For this review, take the finished solid that the model builds, in its own axes (mm). Round coordinates to 2 decimals unless told otherwise and drop trailing zeros. Order: outer loops, then holes, each group sorted by start corner. A loop starts at its lowest first (then second) coordinate and runs counter-clockwise, first axis right, second up. Notation, with made-up numbers: M 77.25,24 L 130.25,24 A18 cw 130.25,41 Z; hole C -26.5,62.5 d6. An arc over 180 degrees is marked long. Use a Markdown table: item, result.
from build123d import *

# Parameters (mm, degrees)
SKETCH_1_W               = 86
SKETCH_1_H               = 86
EXTRUDE_1_DEPTH          = 2
FILLET_3_R               = 14
CUT_EXTRUDE_1_DEPTH      = 61.844062981
CUT_EXTRUDE_1_DEPTH_BACK = 61.844062981
SKETCH_2_R               = 5.5


with BuildPart() as part:
    # 草图1 → 凸台-拉伸1 (new body)
    with BuildSketch(Plane(origin=(0, 0, 0), x_dir=(1, 0, 0), z_dir=(0, 1, 0))):
        Rectangle(SKETCH_1_W, SKETCH_1_H)
    extrude(amount=EXTRUDE_1_DEPTH)

    # 圆角3
    fillet_3_edges = [part.edges().sort_by_distance(p)[0] for p in [
        (43, 1, 43),
        (-43, 1, 43),
        (-43, 1, -43),
        (43, 1, -43),
    ]]
    fillet(fillet_3_edges, radius=FILLET_3_R)

    # 草图2 → 切除-拉伸1 (cut, two sides: drawn at the far end of the back side and taken through both)
    with BuildSketch(Plane(origin=(0, 2, 0), x_dir=(1, 0, 0), z_dir=(0, 1, 0)).offset(-CUT_EXTRUDE_1_DEPTH_BACK)):
        with Locations(Location((-29, 29, 0), (0, 0, 270))):
            Circle(SKETCH_2_R)
        with Locations(Location((-29, -29, 0), (0, 0, 270))):
            Circle(SKETCH_2_R)
        with Locations(Location((29, -29, 0), (0, 0, 270))):
            Circle(SKETCH_2_R)
        with Locations(Location((29, 29, 0), (0, 0, 270))):
            Circle(SKETCH_2_R)
    extrude(amount=CUT_EXTRUDE_1_DEPTH + CUT_EXTRUDE_1_DEPTH_BACK, mode=Mode.SUBTRACT)


solid = part.part
Q1. Draft analysis for pull direction Z (two halves, no side actions). For faces 1 (the cylindrical face through (-39, 1, -38.8)), 2 (the flat face through (-1, 2, -1)), 3 (the cylindrical face through (32.72, 0.99, 24.95)), state which applies: pulls with the +Z half, pulls with the -Z half, needs draft (parallel to the pull), parting line crosses it, or undercut.
Determined:
| item | result |
|---|---|
| face 1 | pulls with the -Z half |
| face 2 | needs draft |
| face 3 | undercut |
Q2. Add section C-C (y = 1.7). Write out the cut boundary in (x, z), then the cut area to 3 significant figures.
Determined:
| item | result |
|---|---|
| outline | M -43,-29 A14 ccw -29,-43 L 29,-43 A14 ccw 43,-29 L 43,29 A14 ccw 29,43 L -29,43 A14 ccw -43,29 Z; hole C -29,-29 d11; hole C -29,29 d11; hole C 29,-29 d11; hole C 29,29 d11 |
| area | 6,850 mm^2 |
Q3. Wall thickness on line 1 along X through (y, z) = (1.35, 29); line 2 along Z through (x, y) = (25, 1.8): over which ranges is each line inside the solid? List them lowest first. Write a range as [from, to].
Determined:
| item | result |
|---|---|
| line 1 | x = [-43, -34.5], [-23.5, 23.5], [34.5, 43] |
| line 2 | z = [-43, -32.77], [-25.23, 25.23], [32.77, 43] |
Q4. Add section B-B (x = -33). Write out the cut boundary in (y, z).
Determined:
| item | result |
|---|---|
| outline | M 0,-42.42 L 2,-42.42 L 2,-32.77 L 0,-32.77 Z; M 0,-25.23 L 2,-25.23 L 2,25.23 L 0,25.23 Z; M 0,32.77 L 2,32.77 L 2,42.42 L 0,42.42 Z |
Q5. Add section A-A (z = -30.5). Write out the cut boundary in (x, y).
Determined:
| item | result |
|---|---|
| outline | M -42.92,0 L -34.29,0 L -34.29,2 L -42.92,2 Z; M -23.71,0 L 23.71,0 L 23.71,2 L -23.71,2 Z; M 34.29,0 L 42.92,0 L 42.92,2 L 34.29,2 Z |
